```python
from build123d import *

# Parameters (mm, degrees)
CUT_EXTRUDE1_DEPTH      = 6
CUT_EXTRUDE1_DEPTH_BACK = 27.06372692
SKETCH2_W               = 8
SKETCH2_H               = 13
SKETCH2_H_2             = 12
CUT_EXTRUDE2_DEPTH      = 27.06372692
CUT_EXTRUDE2_DEPTH_BACK = 27.06372692
SKETCH3_R               = 1
CUT_EXTRUDE4_START      = -8.00090426
CUT_EXTRUDE4_DEPTH      = 16.001809118
SKETCH7_R               = 0.5
CUT_EXTRUDE5_DEPTH      = 35.598668513
SKETCH8_W               = 7.99991565
SKETCH8_H               = 7
CUT_EXTRUDE6_DEPTH      = 29.756672237


with BuildPart() as part:
    # Sketch1 → Revolve1 (revolve)
    with BuildSketch(Plane(origin=(0, 0, 0), x_dir=(0, 0, -1), z_dir=(1, 0, 0))):
        with BuildLine():
            Line((0, 22.5), (0, -22.5))
            Line((0, -22.5), (8, -22.5))
            add(Edge.make_bspline(
                [(8, 22.5), (10.604722665, 7.727883705), (8, -22.5)],
                knots=[0, 0, 0, 1, 1, 1], degree=2))
            Line((8, 22.5), (0, 22.5))
        make_face()
    revolve(axis=Axis((0, 22.5, 0), (0, -1, 0)))

    # Sketch2 → Cut-Extrude1 (cut, two sides: drawn at the far end of the back side and taken through both)
    with BuildSketch(Plane(origin=(0, 0, 0), x_dir=(0, 0, -1), z_dir=(1, 0, 0)).offset(-CUT_EXTRUDE1_DEPTH_BACK)):
        with Locations((0, 16)):
            Rectangle(SKETCH2_W, SKETCH2_H)
        with Locations((0, -16.5)):
            Rectangle(SKETCH2_W, SKETCH2_H_2)
    extrude(amount=CUT_EXTRUDE1_DEPTH + CUT_EXTRUDE1_DEPTH_BACK, mode=Mode.SUBTRACT)

    # Sketch3 → Cut-Extrude2 (cut, two sides: drawn at the far end of the back side and taken through both)
    with BuildSketch(Plane.XY.offset(-CUT_EXTRUDE2_DEPTH_BACK)):
        with Locations((0.535898385, 17.5)):
            Circle(SKETCH3_R)
        with Locations(Location((0.535898385, -19.5, 0), (0, 0, 270))):
            Circle(SKETCH3_R)
    extrude(amount=CUT_EXTRUDE2_DEPTH + CUT_EXTRUDE2_DEPTH_BACK, mode=Mode.SUBTRACT)

    # Cut-Extrude4: read off the stored shape, not the designer's step
    # Cut-Extrude4 outline → Cut-Extrude4 (cut)
    with BuildSketch(Plane.XY.offset(CUT_EXTRUDE4_START)):
        with BuildLine():
            add(Edge.make_bspline(
                [(-7.584242009, -15.120735442), (-7.392641047, -17.582704738), (-7.172738471, -20.042359578), (-6.92820323, -22.5)],
                knots=[0.384705374, 0.384705374, 0.384705374, 0.384705374, 1, 1, 1, 1], degree=3))
            Line((-6.92820323, -22.5), (0.391639605, -22.5))
            ThreePointArc((0.391639605, -22.5), (-5.041320751, -20.37221779), (-7.584242009, -15.120735442))
        make_face()
    extrude(amount=CUT_EXTRUDE4_DEPTH, mode=Mode.SUBTRACT)

    # Sketch7 → Cut-Extrude5 (cut, through all)
    with BuildSketch(Plane(origin=(0, 9.5, 0), x_dir=(1, 0, 0), z_dir=(0, 1, 0))):
        with Locations(Location((-3, 0, 0), (0, 0, 270))):
            Circle(SKETCH7_R)
        with Locations(Location((4, 0, 0), (0, 0, 270))):
            Circle(SKETCH7_R)
    extrude(amount=-CUT_EXTRUDE5_DEPTH, mode=Mode.SUBTRACT)

    # Sketch8 → Cut-Extrude6 (cut, through all)
    with BuildSketch(Plane.ZY.offset(-6)):
        with Locations((-4.2175e-05, -19)):
            Rectangle(SKETCH8_W, SKETCH8_H)
    extrude(amount=-CUT_EXTRUDE6_DEPTH, mode=Mode.SUBTRACT)


solid = part.part
```
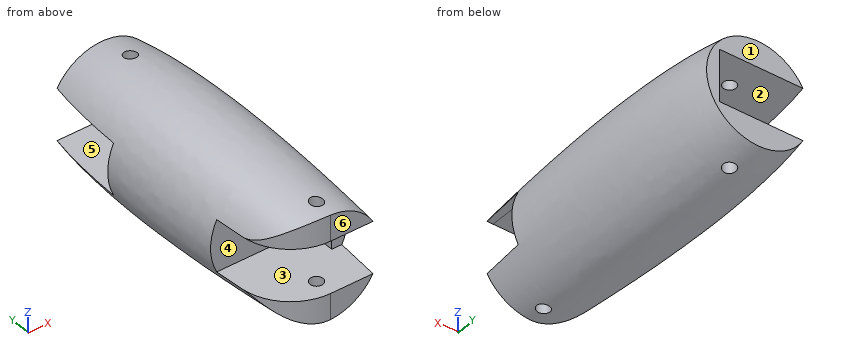
For this review, take the finished solid that the model builds, in its own axes (mm). Face numbers are marked on the shaded views. A direction names the side the tool comes from. Coordinates: 2 decimals unless noted, no trailing zeros.
1. For line 1 (X direction, y = 6.5, z = 0); line 2 (X direction, y = -5, z = -3.75); line 3 (Y direction, x = -4, z = -2.5), list the stretches that pass through material, from the lowest coordinate up.
2. Insertion check: P1, Ø4, axis at y = -6.5, z = -0.5, coming from the -X side; P2, Ø1, axis at x = 3.5, y = -3.5, coming from the -Z side; P3, Ø0.5, axis at x = 6.5, y = -17.5, coming from the -Z side. Each pin has a flat end and moves straight along its axis. Give the tip position at first contact, or say it passes through.
3. Mouldability with a two-part tool opening along Z and no side actions: class the marked faces 4, 5 and 6 as +Z half, -Z half, draft (parallel to the pull), parting line (faces both ways), or undercut.
4. Add section A-A, the plane z = 0. Count the separate pieces of the cut face and the enclosed holes in it, then the cut area to 3 significant figures.
5. For the marked faces 1, 2 and 3, list the 3-axis set-ups (+Z, -Z, +X, -X, +Y, -Y) from which the entire face can be reached by the end or side of a thin tool; tool diameter is ignored.
Result:
1. line 1: x = -9.28 to -3.5, -2.5 to 3.5, 4.5 to 9.28
1. line 2: x = -8.32 to 8.32
1. line 3: y = -10.5 to 9.5
2. P1: stops at x = -9.14
2. P2: stops at z = -8.67
2. P3: stops at z = -5.62
3. face 4: undercut
3. face 5: undercut
3. face 6: draft
4. separate pieces: 3
4. enclosed holes: 0
4. area: 377 mm2
5. face 1: +Z, -Z, +X, -X, +Y
5. face 2: -X, +Y
5. face 3: -X, -Y
